Geometry: final body of the model. Coordinates: model frame, mm. Face numbers are marked on the shaded views. A direction names the side the tool comes from. Give positions to 0.01 mm unless a question says otherwise; leave off trailing zeros. Write each loop counter-clockwise with the first axis right and the second up, starting at its lowest first coordinate (ties: lowest second). Pieces come first, ordered by that corner, then holes.
Q1. Cut plane A-A on x = 0. Return the cut outline in (y, z).
Q2. Draft query along Y for the marked faces 1, 2, 3 and 4. Return one class per face: pulls with the +Y half, pulls with the -Y half, needs draft (parallel to the pull), parting line crosses it, or undercut.
Q3. Line query: L1, parallel to Y at x = -2, z = 7.5; L2, parallel to Z at x = -5.75, y = 32; L3, parallel to Y at x = -4.5, z = 2.25. Output: solid intervals per line, ascending.
Q4. Cut plane B-B on z = 10.75. Return the cut outline in (x, y), plus the area to 3 significant figures.
Q5. Pin query (flat end, axial travel): pin 1 (3.5 mm diameter, centred on x = -4, y = 48.5, fed in from +Z); pin 2 (1 mm diameter, centred on y = -32, z = 11, fed in from -X); pin 3 (8 mm diameter, centred on x = -7, y = 30.5, fed in from -Z); pin 4 (2.5 mm diameter, centred on x = -4, y = -38.1, fed in from +Z). Return the tip coordinate at first contact, or that it passes through.
Q6. Cut plane C-C on x = -6. Return the cut outline in (y, z).
Q7. Reachability of the marked faces 5, 6 and 7 from +Z, -Z, +X, -X, +Y, -Y: full face, straight path, thin tool, end or side. Return the list, or none.
```python
from build123d import *

# Parameters (mm, degrees)
SKETCH_W        = 20
SKETCH_H        = 110
PAD_DEPTH       = 28
SKETCH003_R     = 1
POCKET_DEPTH    = 28.001
SKETCH004_W     = 14
SKETCH004_H     = 25
SKETCH004_W_2   = 12.717113
SKETCH004_H_2   = 24.211324
POCKET001_DEPTH = 20.001
SKETCH005_W     = 82
SKETCH005_H     = 26
POCKET002_DEPTH = 17
SKETCH006_R     = 2.4
POCKET003_DEPTH = 5
FILLET_R        = 2
FILLET001_R     = 5


with BuildPart() as part:
    # Sketch → Pad (new body)
    with BuildSketch(Plane.XY):
        Rectangle(SKETCH_W, SKETCH_H)
    extrude(amount=PAD_DEPTH)

    # Sketch003 → Pocket (cut, through all)
    with BuildSketch(Plane(origin=(0, 0, 0), x_dir=(1, 0, 0), z_dir=(0, 0, -1))):
        with Locations((-4, -0.004117)):
            Circle(SKETCH003_R)
        with Locations((-4, 6.346514)):
            Circle(SKETCH003_R)
        with Locations((-4, 12.697146)):
            Circle(SKETCH003_R)
        with Locations((-4, -6.354749)):
            Circle(SKETCH003_R)
        with Locations((-4, 19.047777)):
            Circle(SKETCH003_R)
        with Locations((-4, 25.398409)):
            Circle(SKETCH003_R)
        with Locations((-4, 31.74904)):
            Circle(SKETCH003_R)
        with Locations((-4, 38.099672)):
            Circle(SKETCH003_R)
        with Locations((-4, -38.107906)):
            Circle(SKETCH003_R)
        with Locations((-4, -12.70538)):
            Circle(SKETCH003_R)
        with Locations((-4, -19.056012)):
            Circle(SKETCH003_R)
        with Locations((-4, -25.406643)):
            Circle(SKETCH003_R)
        with Locations((-4, -31.757274)):
            Circle(SKETCH003_R)
    extrude(amount=-POCKET_DEPTH, mode=Mode.SUBTRACT)

    # Sketch004 → Pocket001 (cut, through all)
    with BuildSketch(Plane.YZ.offset(10)):
        with Locations((-52, 16.5)):
            Rectangle(SKETCH004_W, SKETCH004_H)
        with Locations((51.358556, 16.894338)):
            Rectangle(SKETCH004_W_2, SKETCH004_H_2)
    extrude(amount=-POCKET001_DEPTH, mode=Mode.SUBTRACT)

    # Sketch005 → Pocket002 (cut)
    with BuildSketch(Plane(origin=(-10, 0, 0), x_dir=(0, -1, 0), z_dir=(-1, 0, 0))):
        with Locations((0, 12)):
            Rectangle(SKETCH005_W, SKETCH005_H)
    extrude(amount=-POCKET002_DEPTH, mode=Mode.SUBTRACT)

    # Sketch006 → Pocket003 (cut)
    with BuildSketch(Plane.XY.offset(4.788676)):
        with Locations((0, 50)):
            Circle(SKETCH006_R)
        with Locations((0, -50)):
            Circle(SKETCH006_R)
    extrude(amount=-POCKET003_DEPTH, mode=Mode.SUBTRACT)

    # Fillet
    fillet_edges = [part.edges().sort_by_distance(p)[0] for p in [
        (10, -45, 16),
        (10, 0, 28),
        (10, 45, 16.394338),
        (0, 45, 28),
        (0, -45, 28),
    ]]
    fillet(fillet_edges, radius=FILLET_R)

    # Fillet001
    fillet001_edges = [part.edges().sort_by_distance(p)[0] for p in [
        (10, 55, 2.394338),
        (-10, 55, 2.394338),
        (-10, -55, 2),
        (10, -55, 2),
    ]]
    fillet(fillet001_edges, radius=FILLET001_R)


solid = part.part
```
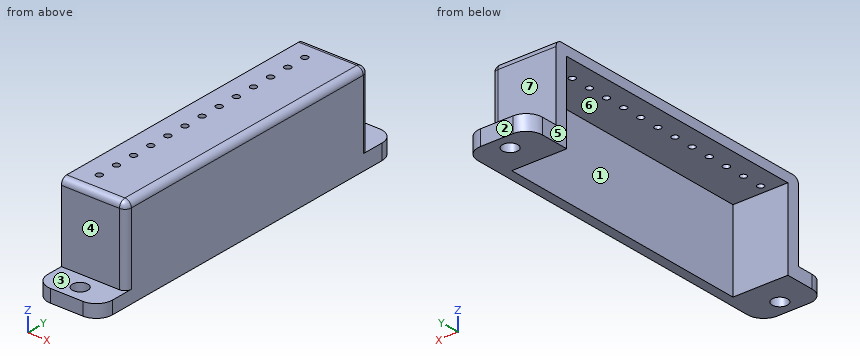
Data:
1. outline: (-55, 0) - (-52.4, 0) - (-52.4, 4) - (-55, 4) - close; (-47.6, 0) - (-41, 0) - (-41, 25) - (41, 25) - (41, 0) - (47.6, 0) - (47.6, 4.79) - (45, 4.79) - (45, 26) arc R2 ccw to (43, 28) - (-43, 28) arc R2 ccw to (-45, 26) - (-45, 4) - (-47.6, 4) - close; (52.4, 0) - (55, 0) - (55, 4.79) - (52.4, 4.79) - close
2. face 1: undercut
2. face 2: pulls with the +Y half
2. face 3: needs draft
2. face 4: pulls with the -Y half
3. L1: y = -45 to -41, 41 to 45
3. L2: z = 25 to 28
3. L3: y = -55 to -41, 41 to 55
4. outline: (-10, -45) - (8, -45) arc R2 ccw to (10, -43) - (10, 43) arc R2 ccw to (8, 45) - (-10, 45) - (-10, 41) - (7, 41) - (7, -41) - (-10, -41) - close
4. area: 404 mm2
5. pin 1: stops at z = 4.79
5. pin 2: stops at x = 7
5. pin 3: stops at z = 25
5. pin 4: stops at z = 28
6. outline: (-54.9, 0) - (-41, 0) - (-41, 25) - (41, 25) - (41, 0) - (54.9, 0) - (54.9, 4.79) - (45, 4.79) - (45, 26) arc R2 ccw to (43, 28) - (-43, 28) arc R2 ccw to (-45, 26) - (-45, 4) - (-54.9, 4) - close
7. face 5: +Z, -Z, -X, +Y, -Y
7. face 6: -Z, -X
7. face 7: +Z, +X, -X, +Y
